Model file for the job. Use its own axes, mm. Give positions to 0.01 mm unless a question says otherwise; leave off trailing zeros. Write each loop counter-clockwise with the first axis right and the second up, starting at its lowest first coordinate (ties: lowest second). Pieces come first, ordered by that corner, then holes.
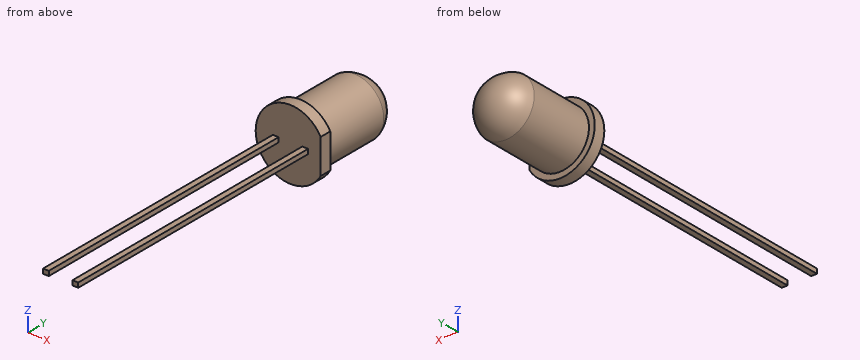
```python
from build123d import *

# Parameters (mm, degrees)
SALIENTE_EXTRUIR2_DEPTH = 1
CROQUIS3_W              = 0.5
CROQUIS3_H              = 0.4
SALIENTE_EXTRUIR3_DEPTH = 24


with BuildPart() as part:
    # Croquis1 → Revolución1 (revolve)
    with BuildSketch(Plane.XY):
        with BuildLine():
            Line((0, 0), (2.5, 0))
            Line((2.5, 0), (2.5, 5.714142843))
            ThreePointArc((2.5, 5.714142843), (1.56576317, 7.075665121), (0, 7.6))
            Line((0, 7.6), (0, 0))
        make_face()
    revolve(axis=Axis((0, 7.6, 0), (0, -1, 0)))

    # Croquis2 → Saliente-Extruir2 (add)
    with BuildSketch(Plane.XZ):
        with BuildLine():
            Line((2.607539428, 1.483488501), (2.607539428, -1.483488501))
            ThreePointArc((2.607539428, -1.483488501), (-3, 0), (2.607539428, 1.483488501))
        make_face()
    extrude(amount=SALIENTE_EXTRUIR2_DEPTH)

    # Croquis3 → Saliente-Extruir3 (add)
    with BuildSketch(Plane.XZ.offset(1)):
        with Locations((1.27, 0)):
            Rectangle(CROQUIS3_W, CROQUIS3_H)
        with Locations((-1.27, 0)):
            Rectangle(CROQUIS3_W, CROQUIS3_H)
    extrude(amount=SALIENTE_EXTRUIR3_DEPTH)


solid = part.part
```
1. Slice it at C-C, the plane z = 1. Write the cut outline in (x, y), and give its area (3 significant figures).
Calculated:
outline: (-2.83, -1) - (2.61, -1) - (2.61, 0) - (2.29, 0) - (2.29, 5.71) arc R2.4 ccw to (-2.29, 5.71) - (-2.29, 0) - (-2.83, 0) - close
area: 37.3 mm2
2. Probe probe 1 along Z at (x, y) = (-1.25, -19.5); probe 2 along Y at (x, z) = (-2.1, 1.5); probe 3 along X at (y, z) = (6, 2). List the from-to ranges inside material, lowest first.
Calculated:
probe 1: z = -0.2 to 0.2
probe 2: y = -1 to 0
probe 3: x = -1.33 to 1.33
3. Slice it at D-D, the plane y = 3. Write the cut outline in (x, z), and give its area (3 significant figures).
Calculated:
outline: circle Ø5 at (0, 0)
area: 19.6 mm2
4. Slice it at A-A, the plane y = -9. Write the cut outline in (x, z).
Calculated:
outline: (-1.52, -0.2) - (-1.02, -0.2) - (-1.02, 0.2) - (-1.52, 0.2) - close; (1.02, -0.2) - (1.52, -0.2) - (1.52, 0.2) - (1.02, 0.2) - close
5. Pin check, flat tips, straight feed: P1, Ø1, axis at y = -19, z = -1.5, coming from the +X side; P2, Ø3, axis at x = 1.5, y = -19.5, coming from the +Z side; P3, Ø3, axis at x = 0, z = 0.5, coming from the -Y side; P4, Ø1.5, axis at x = -1.5, z = 2, coming from the +Y side. Stop position of each tip, or through.
Calculated:
P1: passes through
P2: stops at z = 0.2
P3: stops at y = -25
P4: stops at y = 6.92
6. Slice it at B-B, the plane x = 0. Write the cut outline in (y, z), and give its area (3 significant figures).
Calculated:
outline: (-1, -3) - (0, -3) - (0, -2.5) - (5.71, -2.5) arc R2.6 ccw to (5.71, 2.5) - (0, 2.5) - (0, 3) - (-1, 3) - close
area: 41.5 mm2
